```python
from build123d import *

# Parameters (mm, degrees)
PAD_DEPTH    = 6.2
SKETCH001_W  = 7.7
SKETCH001_H  = 0.2
PAD001_DEPTH = 1.5
PAD002_DEPTH = 3.85
SKETCH003_W  = 0.2
SKETCH003_H  = 4
PAD003_DEPTH = 0.75


with BuildPart() as part:
    # Sketch → Pad (new body)
    with BuildSketch(Plane.YZ):
        with BuildLine():
            ThreePointArc((-3.572464, 9.569314), (-5.05, 6), (-3.572464, 2.430686))
            Line((-3.572464, 0.2), (-3.572464, 2.430686))
            Line((3.572464, 0.2), (-3.572464, 0.2))
            Line((3.572464, 2.430686), (3.572464, 0.2))
            ThreePointArc((3.572464, 2.430686), (5.05, 6), (3.572464, 9.569314))
            ThreePointArc((4.350625, 11.446788), (3.33445, 10.767964), (3.572464, 9.569314))
            ThreePointArc((4.350625, 11.246788), (4.450625, 11.346788), (4.350625, 11.446788))
            ThreePointArc((4.350625, 11.246788), (3.519209, 10.691386), (3.713948, 9.710673))
            ThreePointArc((3.85, 2.430686), (5.249083, 6.098098), (3.713948, 9.710673))
            Line((3.85, 2.430686), (3.85, 0))
            Line((-3.85, 0), (3.85, 0))
            Line((-3.85, 2.430686), (-3.85, 0))
            ThreePointArc((-3.713948, 9.710673), (-5.249083, 6.098098), (-3.85, 2.430686))
            ThreePointArc((-3.713948, 9.710673), (-3.519209, 10.691387), (-4.350626, 11.246788))
            ThreePointArc((-4.350626, 11.446788), (-4.450626, 11.346788), (-4.350626, 11.246788))
            ThreePointArc((-3.572464, 9.569314), (-3.33445, 10.767964), (-4.350626, 11.446788))
        make_face()
    extrude(amount=PAD_DEPTH)

    # Sketch001 → Pad001 (join)
    with BuildSketch(Plane.YZ):
        with Locations((0, 0.1)):
            Rectangle(SKETCH001_W, SKETCH001_H)
    extrude(amount=-PAD001_DEPTH)

    # Sketch002 → Pad002 (join, symmetric)
    with BuildSketch(Plane.XZ):
        with BuildLine():
            Line((-1.5, 0.2), (-0.78, 2.2))
            Line((-0.78, 2.2), (-0.78, 9.8))
            Line((-0.78, 9.8), (-1.292938, 10.9))
            ThreePointArc((-1.111677, 10.984524), (-1.244569, 11.032893), (-1.292938, 10.9))
            Line((-0.58, 9.844339), (-1.111677, 10.984524))
            Line((-0.58, 2.2), (-0.58, 9.844339))
            Line((-1.3, 0.2), (-0.58, 2.2))
            Line((-1.3, 0), (-1.3, 0.2))
            Line((-1.5, 0), (-1.3, 0))
            Line((-1.5, 0.2), (-1.5, 0))
        make_face()
    extrude(amount=PAD002_DEPTH, both=True)

    # Sketch003 → Pad003 (join, symmetric)
    with BuildSketch(Plane.XZ):
        with Locations((0.1, -2)):
            Rectangle(SKETCH003_W, SKETCH003_H)
        with Locations((6.1, -2)):
            Rectangle(SKETCH003_W, SKETCH003_H)
    extrude(amount=PAD003_DEPTH, both=True)


solid = part.part
```
Input: part model. Units: mm. Frame: model coordinates. A direction names the side the tool comes from. Round coordinates to 2 decimals unless told otherwise and drop trailing zeros. Loops run counter-clockwise (first coordinate to the right, second up) from the corner with the lowest first, then second, coordinate; pieces in that order, holes last. Notation, with made-up numbers: (-33, 60.25) - (1, 60.25) arc R8 cw to (1, 68.25) - close; hole circle Ø1 at (-19, 6.25). An arc over 180 degrees is marked (long way). One line per item, written item: value. Start each with the question number.
(1) Access query for faces 1 (the flat face through (-0.78, 0, 6)), 2 (the cylindrical face through (3.057, -3.328, 10.751)), 3 (the flat face through (0, 0, -2)). Directions: +Z, -Z, +X, -X, +Y, -Y. A direction counts if a zero-diameter tool reaches every point of the face in a straight line with its end or side. Return the directions, or none.
(2) Draft query along Y for faces 4 (the cylindrical face through (3.06, 3.34, 10.78)), 5 (the flat face through (-0.945, -0.054, 1.186)), 6 (the cylindrical face through (3.057, -3.514, 10.678)). Return one class per face: +Y half, -Y half, draft (parallel to the pull), parting line (faces both ways), or undercut.
(3) Section D-D, the plane y = -1.5. Return loops of the section in (x, z).
(4) Contact query for flat-ended pins moving along their axis: P1, Ø1.6, axis at y = 0, z = -1.5, coming from the -X side; P2, Ø2.5, axis at x = 2, y = 1.5, coming from the -Z side; P3, Ø1.1, axis at x = 2, z = 1.5, coming from the -Y side; P4, Ø3, axis at x = 3.5, y = -3, coming from the +Z side. Output: stop coordinate, or through.
(5) Section C-C, the plane z = 9.25. Return loops of the section in (x, y), plus the area to 3 significant figures.
(6) Ray query, line 1 (Y direction, x = 0.25, z = 0.75); line 2 (Y direction, x = 2.5, z = 6); line 3 (Z direction, x = 3.5, y = -1). Return the intervals inside material, ascending. Write a range as [from, to].
(7) Section B-B, the plane x = 2. Return loops of the section in (y, z).
(8) Section A-A, the plane z = -3. Return loops of the section in (x, y).
Results below:
1. face 1: -X, +Y, -Y
1. face 2: +X
1. face 3: -Z, -X, +Y, -Y
2. face 4: undercut
2. face 5: draft
2. face 6: -Y half
3. outline: (-1.5, 0) - (6.2, 0) - (6.2, 0.2) - (-1.3, 0.2) - (-0.58, 2.2) - (-0.58, 9.84) - (-1.11, 10.98) arc R0.1 ccw to (-1.29, 10.9) - (-0.78, 9.8) - (-0.78, 2.2) - (-1.5, 0.2) - close
4. P1: x = 0
4. P2: z = 0
4. P3: y = -3.85
4. P4: z = 11.45
5. outline: (-0.78, -3.85) - (-0.58, -3.85) - (-0.58, 3.85) - (-0.78, 3.85) - close; (0, -4.12) - (6.2, -4.12) - (6.2, -3.87) - (0, -3.87) - close; (0, 3.87) - (6.2, 3.87) - (6.2, 4.12) - (0, 4.12) - close
5. area: 4.74 mm^2
6. line 1: [-3.85, -3.57], [3.57, 3.85]
6. line 2: [-5.25, -5.05], [5.05, 5.25]
6. line 3: [0, 0.2]
7. outline: (-4.35, 11.25) arc R0.9 cw to (-3.71, 9.71) arc R5.25 ccw to (-3.85, 2.43) - (-3.85, 0) - (3.85, 0) - (3.85, 2.43) arc R5.25 ccw to (3.71, 9.71) arc R0.9 cw to (4.35, 11.25) arc R0.1 ccw to (4.35, 11.45) arc R1.1 ccw to (3.57, 9.57) arc R5.05 cw to (3.57, 2.43) - (3.57, 0.2) - (-3.57, 0.2) - (-3.57, 2.43) arc R5.05 cw to (-3.57, 9.57) arc R1.1 ccw to (-4.35, 11.45) arc R0.1 ccw to start
8. outline: (0, -0.75) - (0.2, -0.75) - (0.2, 0.75) - (0, 0.75) - close; (6, -0.75) - (6.2, -0.75) - (6.2, 0.75) - (6, 0.75) - close
